```python
from build123d import *

# Parameters (mm, degrees)
F0_W     = 40
F0_H     = 40
F0_R     = 10
F1_DEPTH = 25
F2_DEPTH = 150
F3_R     = 4.99999


# Not quite as in the source:
# - a fillet or chamfer is up to 0.001 mm smaller than in the source, because OpenCascade refuses the exact size


with BuildPart() as f1:
    # F0 (on Top) → F1 (new body)
    with BuildSketch(Plane.XY):
        Rectangle(F0_W, F0_H)
        Circle(F0_R, mode=Mode.SUBTRACT)
    extrude(amount=F1_DEPTH)

    # F0 (on Top) → F2 (join)
    with BuildSketch(Plane.XY):
        Circle(F0_R)
    extrude(amount=F2_DEPTH)

    # F3 (radius 5 in the source; OpenCascade refuses exactly that, so slightly less here)
    f3_edges = [f1.edges().sort_by_distance(p)[0] for p in [
        (20, 0, 0),
        (0, 20, 0),
        (-20, 0, 0),
        (0, -20, 0),
        (-20, 20, 12.5),
        (-20, -20, 12.5),
        (-20, 0, 25),
        (20, -20, 12.5),
        (0, -20, 25),
        (-10, 0, 25),
        (10, 0, 87.5),
        (-10, 0, 150),
        (20, 20, 12.5),
        (20, 0, 25),
        (0, 20, 25),
    ]]
    fillet(f3_edges, radius=F3_R)


solid = f1.part
```
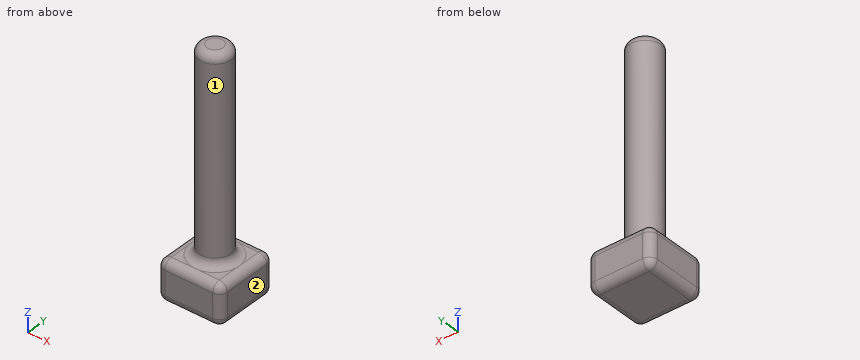
The model under review builds one solid part; all positions refer to its coordinate system, in mm. Face numbers are marked on the shaded views. A direction names the side the tool comes from. Give positions to 0.01 mm unless a question says otherwise; leave off trailing zeros. Write each loop counter-clockwise with the first axis right and the second up, starting at its lowest first coordinate (ties: lowest second). Pieces come first, ordered by that corner, then holes. Notation, with made-up numbers: M 59.25,61.5 L 114.25,61.5 A30 cw 114.25,85.5 Z; hole C 17.5,68 d4. An arc over 180 degrees is marked long. Write item = value, one per line. Start each with the question number.
Q1. For line 1 (Z direction, x = 10, y = 15.5); line 2 (Z direction, x = -7, y = -11.5); line 3 (Y direction, x = -1, z = 34), list the stretches that pass through material, from the lowest coordinate up.
Q2. Clearance check with flat-ended pins moving along their axes: pin 1 (6 mm diameter, centred on x = -3, z = 132, fed in from -Y); pin 2 (5 mm diameter, centred on x = -10.5, z = 64.5, fed in from -Y); pin 3 (8 mm diameter, centred on y = 9.5, z = 120.5, fed in from -X). State where each tip first meets the part, or that it passes through.
Q3. Machinability: for the marked faces 1 and 2, which of the approach directions +Z, -Z, +X, -X, +Y, -Y give a long, thin tool a straight path to every point of the face, cutting with its end or side? Answer none if there is none.
Q4. We need section C-C (z = 115). State the section outline as (x, y) points.
Q5. We need section D-D (x = 17.5). State the section outline as (y, z) points.
Result set:
q1.line_1 = 0.03 to 24.97
q1.line_2 = 0 to 25.24
q1.line_3 = -9.95 to 9.95
q2.pin_1 = -10
q2.pin_2 = -6
q2.pin_3 = -8.35
q3.face_1 = +Z
q3.face_2 = +Z, -Z, +X, +Y, -Y
q4.outline = C 0,0 d20
q5.outline = M -19.33,5 A4.33 ccw -15,0.67 L 15,0.67 A4.33 ccw 19.33,5 L 19.33,20 A4.33 ccw 15,24.33 L -15,24.33 A4.33 ccw -19.33,20 Z
